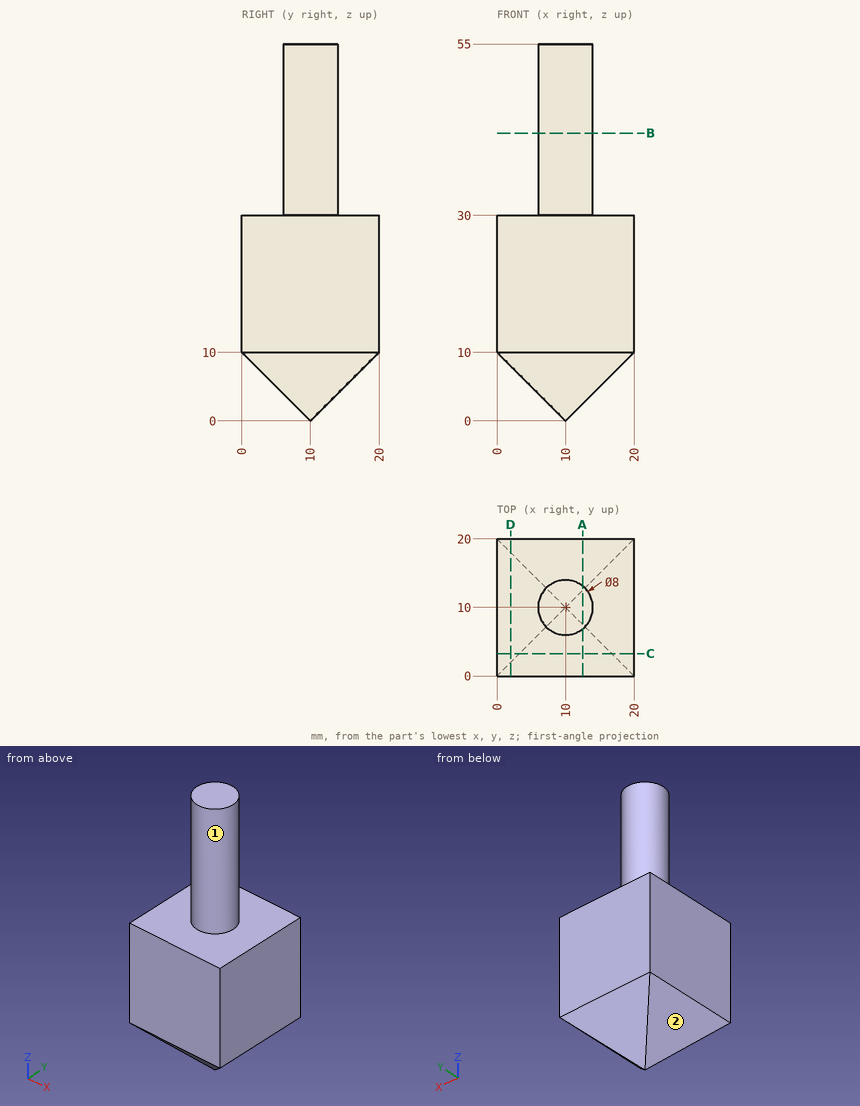
Can you work these out from the drawing? Everything is in mm from the part's minimum corner. A direction names the side the tool comes from. Give positions to 0.01 mm unless a question says otherwise; leave off trailing zeros. Order: outer loops, then holes, each group sorted by start corner. A loop starts at its lowest first (then second) coordinate and runs counter-clockwise, first axis right, second up. Notation, with made-up numbers: M 46.25,11.5 L 80.25,11.5 A11 ccw 80.25,29.5 Z; hole C 72.5,55.5 d5. An arc over 180 degrees is marked long. Use a Markdown table: item, result. Add a question column.
1. For pin 1 Ø6 at (y, z) = (9, 39) entering from -X; pin 2 Ø1.5 at (y, z) = (8, 34) entering from -X; pin 3 Ø5 at (x, z) = (18, 39) entering from +Y; pin 4 Ø1.5 at (x, y) = (7.5, 4) entering from +Z, each with a flat end and sliding along its axis, tell me the tip position at first contact or that it passes through.
2. Suppose I cut it at C-C (y = 3.25). List the corners of the cut face in (x, z) for me.
3. Suppose I cut it at A-A (x = 12.5). List the corners of the cut face in (y, z) for me.
4. I need wall thicknesses on probe 1 along Z at (x, y) = (8.5, 16); probe 2 along Y at (x, z) = (13, 4); probe 3 along Z at (x, y) = (3.25, 15.5). Which ranges of each line are inside material? Lowest first, please. Write a range as from..to.
5. Suppose I cut it at B-B (z = 42). List the corners of the cut face in (x, y) for me, and give its area (3 significant figures).
6. On a 3-axis mill with a long thin cutter (end or side, diameter ignored), from which of +Z, -Z, +X, -X, +Y, -Y can I reach the whole of each face in a straight line? I mean the marked faces 1 and 2. Say none if no direction works.
7. Suppose I cut it at D-D (x = 2). List the corners of the cut face in (y, z) for me.
Results list:
| question | item | result |
|---|---|---|
| 1 | pin 1 | stops at x = 6 |
| 1 | pin 2 | stops at x = 6.2 |
| 1 | pin 3 | passes through |
| 1 | pin 4 | stops at z = 30 |
| 2 | outline | M 0,10 L 3.25,6.75 L 16.75,6.75 L 20,10 L 20,30 L 0,30 Z |
| 3 | outline | M 0,10 L 7.5,2.5 L 12.5,2.5 L 20,10 L 20,30 L 13.12,30 L 13.12,55 L 6.88,55 L 6.88,30 L 0,30 Z |
| 4 | probe 1 | z = 6..30 |
| 4 | probe 2 | y = 6..14 |
| 4 | probe 3 | z = 6.75..30 |
| 5 | outline | C 10,10 d8 |
| 5 | area | 50.3 mm² |
| 6 | face 1 | +Z |
| 6 | face 2 | -Z, -X, +Y, -Y |
| 7 | outline | M 0,10 L 2,8 L 18,8 L 20,10 L 20,30 L 0,30 Z |
